```python
from build123d import *

# Parameters (mm, degrees)
BOSS_EXTRUDE1_DEPTH = 38.1
SKETCH2_R           = 3.571875
CUT_EXTRUDE1_DEPTH  = 559.820020083


with BuildPart() as part:
    # Sketch1 → Boss-Extrude1 (new body)
    with BuildSketch(Plane(origin=(0, 0, 0), x_dir=(0, 0, -1), z_dir=(1, 0, 0))):
        Polygon((0, 88.9), (550.386223343, 88.9), (488.137773196, 0), (0, 0), align=None)
    extrude(amount=BOSS_EXTRUDE1_DEPTH)

    # Sketch2 → Cut-Extrude1 (cut, through all)
    with BuildSketch(Plane(origin=(38.1, 0, 0), x_dir=(0, 0, -1), z_dir=(1, 0, 0))):
        with Locations((23.8125, 44.45)):
            Circle(SKETCH2_R)
        with Locations((465.1375, 44.45)):
            Circle(SKETCH2_R)
    extrude(amount=-CUT_EXTRUDE1_DEPTH, mode=Mode.SUBTRACT)


solid = part.part
```
Geometry check sheet. Reference: the model listing, model coordinates, mm. Round coordinates to 2 decimals unless told otherwise and drop trailing zeros. Loops run counter-clockwise (first coordinate to the right, second up) from the corner with the lowest first, then second, coordinate; pieces in that order, holes last. Notation, with made-up numbers: M 69,82.25 L 120,82.25 A15 cw 120,108.25 Z; hole C 51,-15 d9. An arc over 180 degrees is marked long. Return JSON: item names as keys, results as strings. Group by question number.
(1) Section check C-C, the plane y = 60. Enter the section's corners in (x, z), and give its area (3 significant figures).
(2) Section check A-A, the plane x = 29.5. Enter the section's corners in (y, z).
(3) Section check B-B, the plane y = 22. Enter the section's corners in (x, z), and give its area (3 significant figures).
(4) Scan lines: line 1 along Z through (x, y) = (8.5, 54); line 2 along Z through (x, y) = (21, 57); line 3 along Y through (x, z) = (21.5, -504). Record each from-to range of solid material in increasing order. Write a range as [from, to].
(5) Go/stop test with flat-tipped pins: pin 1 (6 mm diameter, centred on x = 10.5, y = 68, fed in from -Z); pin 2 (1 mm diameter, centred on x = 21.5, y = 51.5, fed in from -Z); pin 3 (8 mm diameter, centred on x = 11, y = 9.5, fed in from -Z). Record where each tip stops, or that it passes through.
Data:
{
 "1": {"outline": "M 0,-530.15 L 38.1,-530.15 L 38.1,0 L 0,0 Z", "area": "20,200 mm²"},
 "2": {"outline": "M 0,-488.14 L 88.9,-550.39 L 88.9,0 L 0,0 Z; hole C 44.45,-465.14 d7.14; hole C 44.45,-23.81 d7.14"},
 "3": {"outline": "M 0,-503.54 L 38.1,-503.54 L 38.1,0 L 0,0 Z", "area": "19,200 mm²"},
 "4": {"line 1": "[-525.95, 0]", "line 2": "[-528.05, 0]", "line 3": "[22.65, 88.9]"},
 "5": {"pin 1": "z = -537.85", "pin 2": "z = -524.55", "pin 3": "z = -497.59"}
}
